Input: dimensioned drawing with shaded views. Units: mm. Origin: part minimum x, y, z. Round coordinates to 2 decimals unless told otherwise and drop trailing zeros. Order: outer loops, then holes, each group sorted by start corner. A loop starts at its lowest first (then second) coordinate and runs counter-clockwise, first axis right, second up. Notation, with made-up numbers: M -23,59 L 18,59 A17 ccw 18,90 Z; hole C 78,12.5 d1. An arc over 180 degrees is marked long. Use CSV: the item, a comma, the result in double quotes. Start each with the question number.
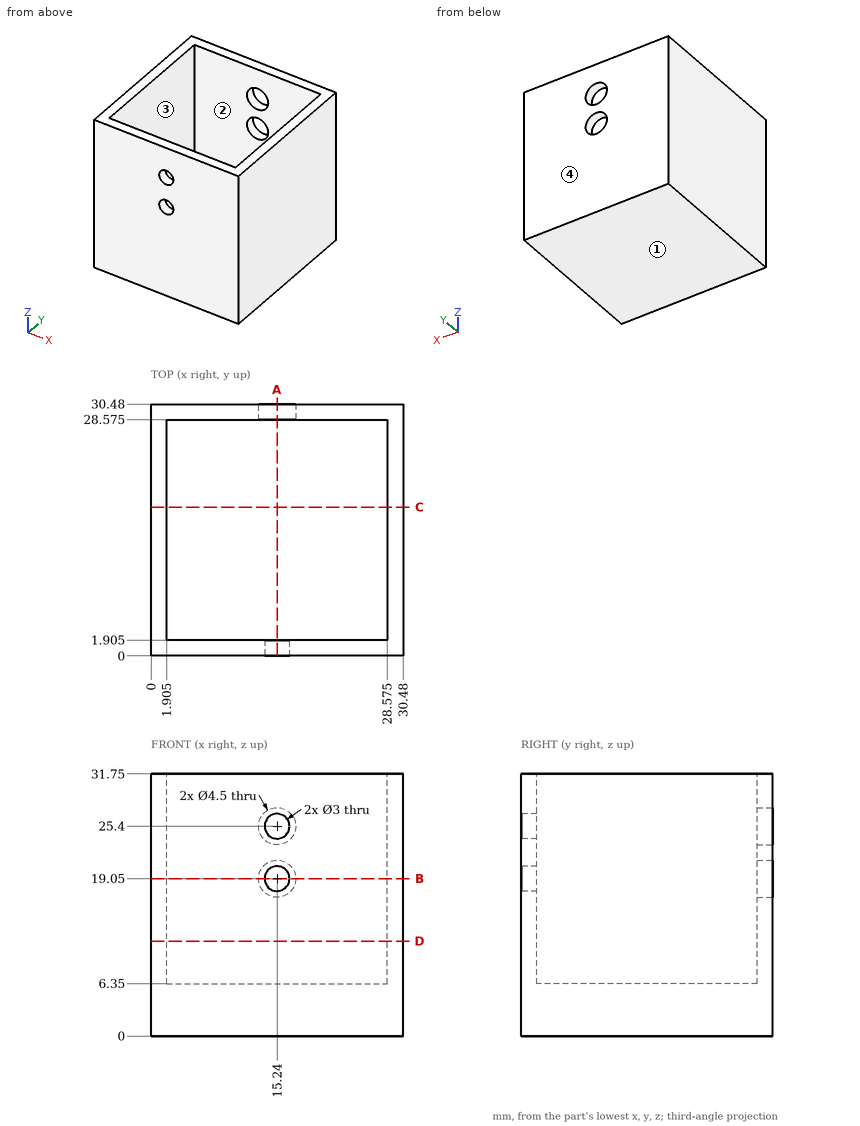
(1) Line query: line 1 along Z through (x, y) = (15.24, 1.5); line 2 along X through (y, z) = (2, 8.5) (3 decimals); line 3 along X through (y, z) = (29.75, 19.05). Output: solid intervals per line, ascending.
(2) Section B-B on z = 19.05. Return loops of the section in (x, y) (3 decimals).
(3) Section A-A on x = 15.24. Return loops of the section in (y, z) (3 decimals).
(4) Draft query along Y for the marked faces 1, 2, 3 and 4. Return one class per face: pulls with the +Y half, pulls with the -Y half, needs draft (parallel to the pull), parting line crosses it, or undercut.
(5) Contact query for a flat-ended pin moving along its axis: P1, Ø8, axis at x = 13, y = 19, coming from the +Z side. Output: stop coordinate, or through.
(6) Section C-C on y = 18. Return loops of the section in (x, z) (3 decimals), plus the area to 3 significant figures.
(7) Section D-D on z = 11.5. Return loops of the section in (x, y) (3 decimals), plus the area to 3 significant figures.
Results below:
1,line 1,"z = 0 to 17.55, 20.55 to 23.9, 26.9 to 31.75"
1,line 2,"x = 0 to 1.905, 28.575 to 30.48"
1,line 3,"x = 0 to 12.99, 17.49 to 30.48"
2,outline,"M 0,0 L 13.74,0 L 13.74,1.905 L 1.905,1.905 L 1.905,28.575 L 12.99,28.575 L 12.99,30.48 L 0,30.48 Z; M 16.74,0 L 30.48,0 L 30.48,30.48 L 17.49,30.48 L 17.49,28.575 L 28.575,28.575 L 28.575,1.905 L 16.74,1.905 Z"
3,outline,"M 0,0 L 30.48,0 L 30.48,16.8 L 28.575,16.8 L 28.575,6.35 L 1.905,6.35 L 1.905,17.55 L 0,17.55 Z; M 0,20.55 L 1.905,20.55 L 1.905,23.9 L 0,23.9 Z; M 0,26.9 L 1.905,26.9 L 1.905,31.75 L 0,31.75 Z; M 28.575,21.3 L 30.48,21.3 L 30.48,23.15 L 28.575,23.15 Z; M 28.575,27.65 L 30.48,27.65 L 30.48,31.75 L 28.575,31.75 Z"
4,face 1,"needs draft"
4,face 2,"undercut"
4,face 3,"undercut"
4,face 4,"pulls with the +Y half"
5,P1,"stops at z = 6.35"
6,outline,"M 0,0 L 30.48,0 L 30.48,31.75 L 28.575,31.75 L 28.575,6.35 L 1.905,6.35 L 1.905,31.75 L 0,31.75 Z"
6,area,"290 mm2"
7,outline,"M 0,0 L 30.48,0 L 30.48,30.48 L 0,30.48 Z; hole M 1.905,1.905 L 28.575,1.905 L 28.575,28.575 L 1.905,28.575 Z"
7,area,"218 mm2"
